```python
from build123d import *

# Parameters (mm, degrees)
SKETCH_R        = 1.5
PAD_DEPTH       = 14.5
SKETCH001_R     = 3
POCKET_DEPTH    = 9.5
SKETCH002_R     = 2.5
POCKET001_DEPTH = 9
FILLET_R        = 1.3


with BuildPart() as part:
    # Sketch → Pad (new body)
    with BuildSketch(Plane.XY):
        Polygon((-20, 0), (0, 25), (20, 0), (0, -25), align=None)
        with Locations((0, 20)):
            Circle(SKETCH_R, mode=Mode.SUBTRACT)
        with Locations((0, -20)):
            Circle(SKETCH_R, mode=Mode.SUBTRACT)
        with Locations((-15, 0)):
            Circle(SKETCH_R, mode=Mode.SUBTRACT)
        Circle(SKETCH_R, mode=Mode.SUBTRACT)
        with Locations((15, 0)):
            Circle(SKETCH_R, mode=Mode.SUBTRACT)
    extrude(amount=PAD_DEPTH)

    # Sketch001 (on Face10 of Pad) → Pocket (cut)
    with BuildSketch(Plane(origin=(0, 0, 0), x_dir=(1, 0, 0), z_dir=(0, 0, -1))):
        with BuildLine():
            ThreePointArc((-15, 9.5), (-24.5, 0), (-15, -9.5))
            Line((-15, -9.5), (15, -9.5))
            ThreePointArc((15, -9.5), (24.5, 0), (15, 9.5))
            Line((-15, 9.5), (15, 9.5))
        make_face()
        with Locations((-15, 0)):
            Circle(SKETCH001_R, mode=Mode.SUBTRACT)
        Circle(SKETCH001_R, mode=Mode.SUBTRACT)
        with Locations((15, 0)):
            Circle(SKETCH001_R, mode=Mode.SUBTRACT)
    extrude(amount=-POCKET_DEPTH, mode=Mode.SUBTRACT)

    # Sketch002 (on Face20 of Pocket) → Pocket001 (cut)
    with BuildSketch(Plane(origin=(0, 0, 0), x_dir=(1, 0, 0), z_dir=(0, 0, -1))):
        Polygon((-20, 25), (-20, -25), (-5, -25), (-5, -9.5), (5, -9.5), (5, -25), (20, -25), (20, 25), (5, 25), (5, 9.5), (-5, 9.5), (-5, 25), align=None)
        Circle(SKETCH002_R, mode=Mode.SUBTRACT)
        with Locations((-15, 0)):
            Circle(SKETCH002_R, mode=Mode.SUBTRACT)
        with Locations((15, 0)):
            Circle(SKETCH002_R, mode=Mode.SUBTRACT)
    extrude(amount=-POCKET001_DEPTH, mode=Mode.SUBTRACT)

    # Fillet
    fillet_edges = [part.edges().sort_by_distance(p)[0] for p in [
        (10, -12.5, 14.5),
        (-10, -12.5, 14.5),
        (-10, 12.5, 14.5),
        (10, 12.5, 14.5),
        (0, -25, 7.25),
        (5, -18.75, 4.5),
        (-5, -18.75, 4.5),
        (20, 0, 12),
        (-20, 0, 12),
        (-5, 18.75, 4.5),
        (0, 25, 7.25),
        (5, 18.75, 4.5),
        (-5, -9.5, 4.5),
        (5, -9.5, 4.5),
        (5, 9.5, 4.5),
        (-5, 9.5, 4.5),
    ]]
    fillet(fillet_edges, radius=FILLET_R)


solid = part.part
```
Source: CAD feature listing. Evaluate the final solid. Frame: model axes, mm. A direction names the side the tool comes from. Round coordinates to 2 decimals unless told otherwise and drop trailing zeros. Write each loop counter-clockwise with the first axis right and the second up, starting at its lowest first coordinate (ties: lowest second). Pieces come first, ordered by that corner, then holes. Notation, with made-up numbers: M -29.5,34.25 L -21.5,34.25 A29 ccw -21.5,56.25 Z; hole C 55.25,49.5 d6. An arc over 180 degrees is marked long. Use CSV: the item, a comma, the result in double quotes. Start each with the question number.
Q1. Pull-direction query (Y, two-part tool) for faces 5 (the face through (-9.765, 12.2, 14.109)), 6 (the face through (15, -2, 0)), 7 (the face through (-0.195, -18.513, 7.148)); classes: +Y half, -Y half, draft (parallel to the pull), parting line (faces both ways), or undercut.
Q2. Line query: line 1 (Y direction, x = -15, z = 4.5); line 2 (Y direction, x = 15, z = 9.25); line 3 (Z direction, x = -12.5, y = -7.5). Output: solid intervals per line, ascending. Write a range as from..to.
Q3. Cut plane B-B on z = 12.25. Output: boundary loops of the cut face in (x, y).
Q4. Cut plane A-A on z = 7.75. Count the separate pieces of the cut face and the enclosed holes in it, plus the area to 3 significant figures.
Q5. Access query for faces 1 (the face through (-4.63, -9.89, 4.56)), 2 (the face through (-5, -14, 4)), 3 (the face through (0, 9.5, 5)), 4 (the face through (-0.54, 2.44, 4.44)). Directions: +Z, -Z, +X, -X, +Y, -Y. A direction counts if a zero-diameter tool reaches every point of the face in a straight line with its end or side. Return the directions, or none.
Q6. First-contact query: P1, Ø2, axis at y = -16, z = 3.5, coming from the -X side; P2, Ø12, axis at x = -12.5, y = -17.5, coming from the -Z side; P3, Ø5, axis at x = 4, z = 3.5, coming from the -Y side (3 decimals). Flat tips, straight axial feed; report the tip coordinate or a pass-through.
Results found:
1,face 5,"+Y half"
1,face 6,"draft"
1,face 7,"undercut"
2,line 1,"-2.5..-1.5, 1.5..2.5"
2,line 2,"-3..-1.5, 1.5..3"
2,line 3,"9.5..14.49"
3,outline,"M -19.35,-0.81 L -1.02,-23.73 A1.3 ccw 1.02,-23.73 L 19.35,-0.81 A1.3 ccw 19.35,0.81 L 1.02,23.73 A1.3 ccw -1.02,23.73 L -19.35,0.81 A1.3 ccw Z; hole C -15,0 d3; hole C 0,-20 d3; hole C 0,0 d3; hole C 0,20 d3; hole C 15,0 d3"
4,separate pieces,"5"
4,enclosed holes,"5"
4,area,"268 mm^2"
5,face 1,"-Z, -X"
5,face 2,"-Z, -X, +Y, -Y"
5,face 3,"-Z, +X, -X"
5,face 4,"-Z"
6,P1,"x = -5"
6,P2,"z = 9"
6,P3,"y = -23.125"
